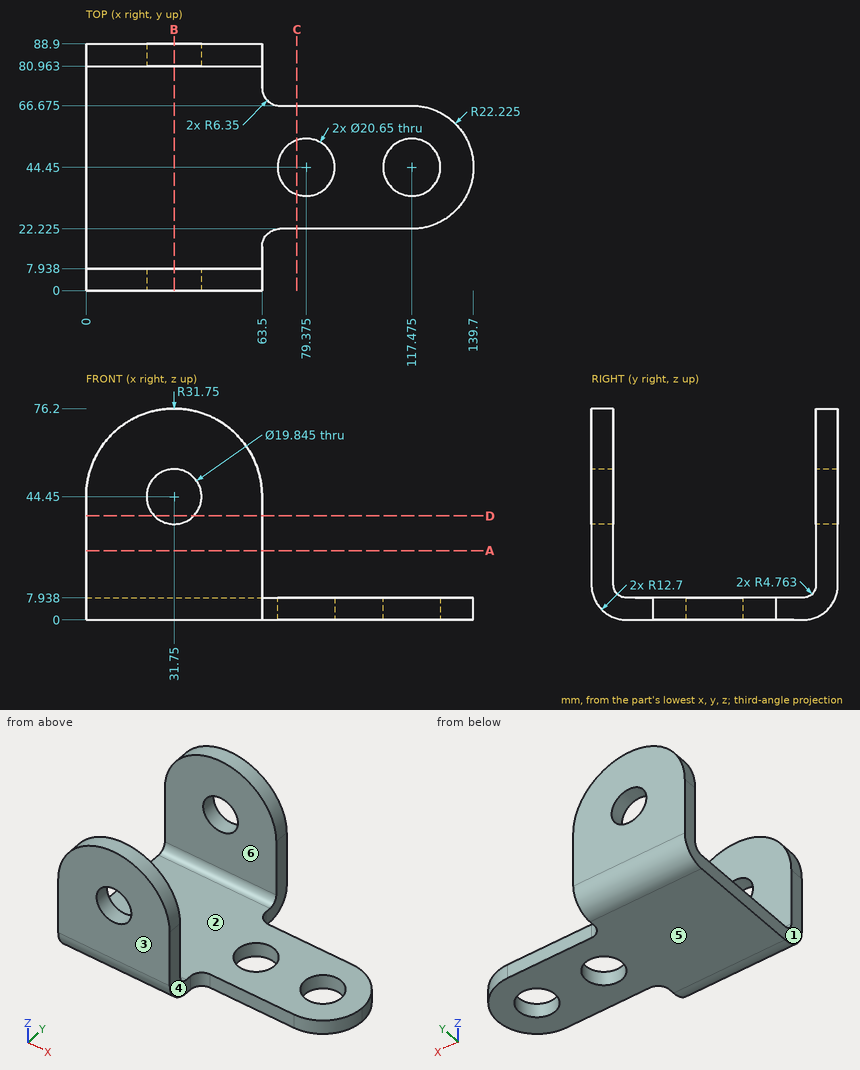
The drawing under review shows one solid part. Ordinate dimensions are in mm from its lowest x, y, z. A direction names the side the tool comes from. Coordinates: 2 decimals unless noted, no trailing zeros. Write each loop counter-clockwise with the first axis right and the second up, starting at its lowest first coordinate (ties: lowest second). Pieces come first, ordered by that corner, then holes.
1) Add section C-C (x = 76). Write out the cut boundary in (y, z) (1 decimal).
2) Add section B-B (x = 31.75). Write out the cut boundary in (y, z) (1 decimal).
3) Add section A-A (z = 25). Write out the cut boundary in (x, y).
4) Mouldability with a two-part tool opening along Y and no side actions: class the marked faces 1, 2 and 3 as +Y half, -Y half, draft (parallel to the pull), parting line (faces both ways), or undercut.
5) Machinability: for the marked faces 4, 5 and 6, which of the approach directions +Z, -Z, +X, -X, +Y, -Y give a long, thin tool a straight path to every point of the face, cutting with its end or side? Answer none if there is none.
6) Insertion check: pin 1 (4 mm diameter, centred on x = 91.5, z = 5.5, fed in from -Y) (1 decimal); pin 2 (2.5 mm diameter, centred on x = 98, z = 4.5, fed in from +Y) (1 decimal); pin 3 (10 mm diameter, centred on x = 53, z = 48.5, fed in from -Y); pin 4 (5 mm diameter, centred on y = 4, z = 15.5, fed in from +X). Each pin has a flat end and moves straight along its axis. Give the tip position at first contact, or say it passes through.
7) To check wall thickness, follow L1, parallel to X at y = 44, z = 2 (1 decimal); L2, parallel to Y at x = 28, z = 60.5; L3, parallel to Z at x = 13.5, y = 23. State the ranges of each line that lie inside material, in increasing order.
8) Add section D-D (z = 37.5). Write out the cut boundary in (x, y).
Check result:
1. outline: (22.2, 0) - (34.7, 0) - (34.7, 7.9) - (22.2, 7.9) - close; (54.2, 0) - (66.7, 0) - (66.7, 7.9) - (54.2, 7.9) - close
2. outline: (0, 12.7) arc R12.7 ccw to (12.7, 0) - (76.2, 0) arc R12.7 ccw to (88.9, 12.7) - (88.9, 34.5) - (81, 34.5) - (81, 12.7) arc R4.8 cw to (76.2, 7.9) - (12.7, 7.9) arc R4.8 cw to (7.9, 12.7) - (7.9, 34.5) - (0, 34.5) - close; (0, 54.4) - (7.9, 54.4) - (7.9, 76.2) - (0, 76.2) - close; (81, 54.4) - (88.9, 54.4) - (88.9, 76.2) - (81, 76.2) - close
3. outline: (0, 0) - (63.5, 0) - (63.5, 7.94) - (0, 7.94) - close; (0, 80.96) - (63.5, 80.96) - (63.5, 88.9) - (0, 88.9) - close
4. face 1: draft
4. face 2: undercut
4. face 3: -Y half
5. face 4: +Z, -Z, +X, -Y
5. face 5: -Z, +X, -X, +Y, -Y
5. face 6: +Z, +X, -X
6. pin 1: stops at y = 22.2
6. pin 2: stops at y = 66.7
6. pin 3: stops at y = 0
6. pin 4: stops at x = 63.5
7. L1: x = 0 to 69.1, 89.7 to 107.2, 127.8 to 139.7
7. L2: y = 0 to 7.94, 80.96 to 88.9
7. L3: z = 0 to 7.94
8. outline: (0, 0) - (24.67, 0) - (24.67, 7.94) - (0, 7.94) - close; (0, 80.96) - (24.67, 80.96) - (24.67, 88.9) - (0, 88.9) - close; (38.83, 0) - (63.5, 0) - (63.5, 7.94) - (38.83, 7.94) - close; (38.83, 80.96) - (63.5, 80.96) - (63.5, 88.9) - (38.83, 88.9) - close
